Part print with two shaded views. Sizes in mm from the minimum x, y, z corner. Coordinates: 2 decimals unless noted, no trailing zeros. Order: outer loops, then holes, each group sorted by start corner. A loop starts at its lowest first (then second) coordinate and runs counter-clockwise, first axis right, second up. Notation, with made-up numbers: (89.25, 0) - (145.25, 0) arc R7 cw to (145.25, 11) - close; hole circle Ø7 at (16.25, 3.5). An arc over 180 degrees is marked (long way). Return JSON: item names as keys, results as strings.
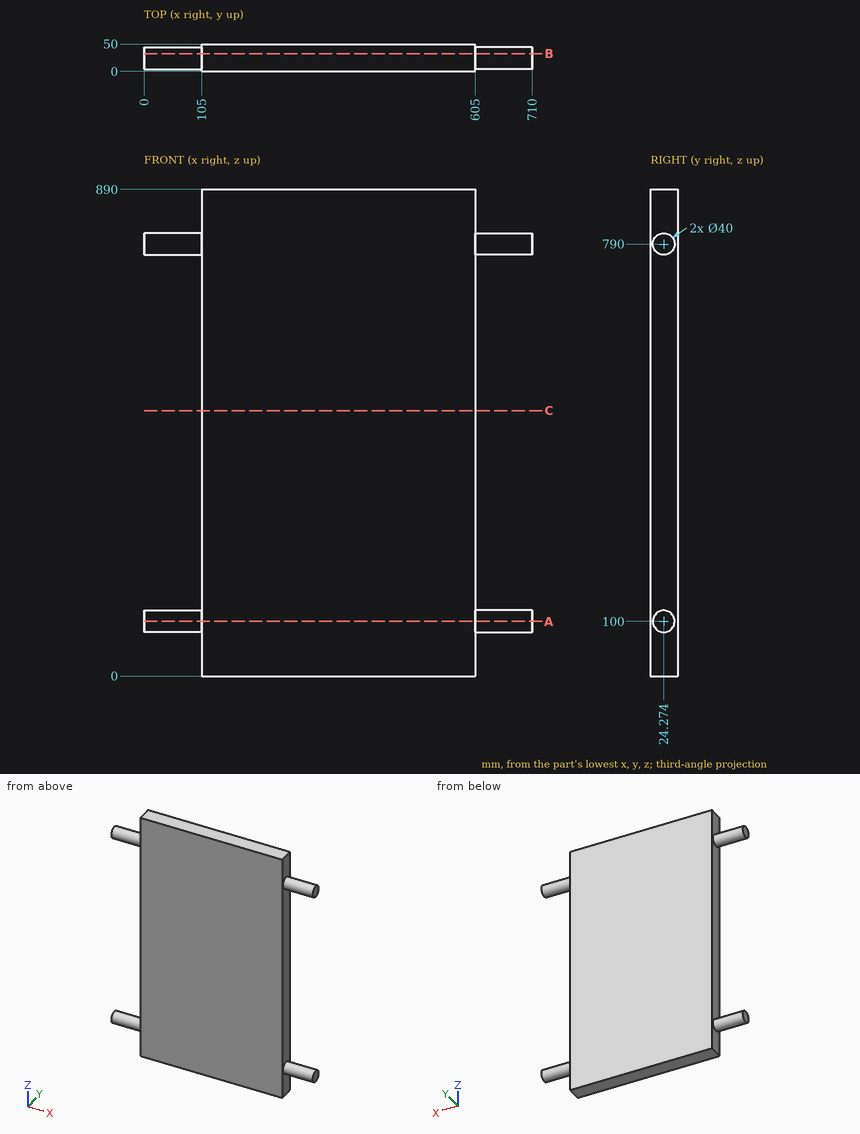
Item 1: Band-saw the part on C-C, the plane z = 485.5. List the corners of the cut face in (x, y).
Findings below:
{"outline": "(105, 0) - (605, 0) - (605, 50) - (105, 50) - close"}
Item 2: Drop flat-ended pins along their axis: P1, Ø4, axis at y = 39, z = 199, coming from the +X side; P2, Ø10, axis at x = 124.5, z = 319.5, coming from the -Y side; P3, Ø25, axis at y = 14, z = 508, coming from the -X side. Give the stop position or say it passes through.
Findings below:
{"P1": "stops at x = 605", "P2": "stops at y = 0", "P3": "stops at x = 105"}
Item 3: Band-saw the part on B-B, the plane y = 32.5. List the corners of the cut face in (x, z).
Findings below:
{"outline": "(0, 81.77) - (105, 81.77) - (105, 0) - (605, 0) - (605, 81.77) - (710, 81.77) - (710, 118.23) - (605, 118.23) - (605, 771.77) - (710, 771.77) - (710, 808.23) - (605, 808.23) - (605, 890) - (105, 890) - (105, 808.23) - (0, 808.23) - (0, 771.77) - (105, 771.77) - (105, 118.23) - (0, 118.23) - close"}
Item 4: Wall check: L1, parallel to X at y = 16, z = 58.5; L2, parallel to Z at x = 629, y = 28; L3, parallel to Z at x = 77, y = 13.5. Give the ranges that are in metal, low to high. Write a range as [from, to].
Findings below:
{"L1": "x = [105, 605]", "L2": "z = [80.35, 119.65], [770.35, 809.65]", "L3": "z = [83.15, 116.85], [773.15, 806.85]"}
Item 5: Band-saw the part on A-A, the plane z = 100. List the corners of the cut face in (x, y).
Findings below:
{"outline": "(0, 4.27) - (105, 4.27) - (105, 0) - (605, 0) - (605, 4.27) - (710, 4.27) - (710, 44.27) - (605, 44.27) - (605, 50) - (105, 50) - (105, 44.27) - (0, 44.27) - close"}
